```python
from build123d import *

# Parameters (mm, degrees)
F1_DEPTH = 1.524
F3_DEPTH = 40.132
F5_DEPTH = 2.794
F8_R     = 1.5875
F9_R     = 1.5875
F10_R    = 1.5875
F11_R    = 1.5875


with BuildPart() as f1:
    # F0 (on Right) → F1 (new body)
    with BuildSketch(Plane.YZ):
        with BuildLine():
            ThreePointArc((26.67, 16.002), (25.7400640303, 18.2470640303), (23.495, 19.177))
            Line((23.495, 19.177), (-23.495, 19.177))
            ThreePointArc((-23.495, 19.177), (-25.7400640303, 18.2470640303), (-26.67, 16.002))
            Line((-26.67, 16.002), (-26.67, -16.002))
            ThreePointArc((-26.67, -16.002), (-25.7400640303, -18.2470640303), (-23.495, -19.177))
            Line((-23.495, -19.177), (23.495, -19.177))
            ThreePointArc((23.495, -19.177), (25.7400640303, -18.2470640303), (26.67, -16.002))
            Line((26.67, -16.002), (26.67, 16.002))
        make_face()
    extrude(amount=F1_DEPTH)

    # F2 (on face) → F3 (join)
    with BuildSketch(Plane(origin=(0, 0, 0), x_dir=(0, -1, 0), z_dir=(-1, 0, 0))):
        with BuildLine():
            ThreePointArc((-23.495, 19.177), (-25.7400640303, 18.2470640303), (-26.67, 16.002))
            Line((-26.67, 16.002), (-26.67, -16.002))
            ThreePointArc((-26.67, -16.002), (-25.7400640303, -18.2470640303), (-23.495, -19.177))
            Line((-23.495, -19.177), (23.495, -19.177))
            ThreePointArc((23.495, -19.177), (25.7400640303, -18.2470640303), (26.67, -16.002))
            Line((26.67, -16.002), (26.67, 16.002))
            ThreePointArc((26.67, 16.002), (25.7400640303, 18.2470640303), (23.495, 19.177))
            Line((23.495, 19.177), (-23.495, 19.177))
        make_face()
        with BuildLine():
            ThreePointArc((25.146, -16.0655), (24.6810320151, -17.1880320151), (23.5585, -17.653))
            Line((23.5585, -17.653), (-23.5585, -17.653))
            ThreePointArc((-23.5585, -17.653), (-24.6810320151, -17.1880320151), (-25.146, -16.0655))
            Line((-25.146, -16.0655), (-25.146, 16.0655))
            ThreePointArc((-25.146, 16.0655), (-24.6810320151, 17.1880320151), (-23.5585, 17.653))
            Line((-23.5585, 17.653), (23.5585, 17.653))
            ThreePointArc((23.5585, 17.653), (24.6810320151, 17.1880320151), (25.146, 16.0655))
            Line((25.146, 16.0655), (25.146, -16.0655))
        make_face(mode=Mode.SUBTRACT)
    extrude(amount=F3_DEPTH)

    # F4 (on face) → F5 (join)
    with BuildSketch(Plane.YZ.offset(1.524)):
        with BuildLine():
            ThreePointArc((-26.67, 12.827), (-22.1798719395, 14.6868719395), (-20.32, 19.177))
            Line((-20.32, 19.177), (-23.495, 19.177))
            ThreePointArc((-23.495, 19.177), (-25.7400640303, 18.2470640303), (-26.67, 16.002))
            Line((-26.67, 16.002), (-26.67, 12.827))
        make_face()
    extrude(amount=F5_DEPTH)


with BuildPart() as f6_1:
    # F6: instance of F1
    add(f1.part.mirror(Plane.XY))


with BuildPart() as f1_1:
    add(f1.part)

    add(f6_1.part)  # F7 merges F6_1
    # F7: F6_1, F1 across plane
    add(f6_1.part.mirror(Plane.XZ))
    add(f1.part.mirror(Plane.XZ))

    # F8
    f8_edges = [f1_1.edges().sort_by_distance(p)[0] for p in [
        (1.524, -26.67, 0),
    ]]
    fillet(f8_edges, radius=F8_R)

    # F9
    f9_edges = [f1_1.edges().sort_by_distance(p)[0] for p in [
        (1.524, 0, -19.177),
    ]]
    fillet(f9_edges, radius=F9_R)

    # F10
    f10_edges = [f1_1.edges().sort_by_distance(p)[0] for p in [
        (1.524, 26.67, 0),
    ]]
    fillet(f10_edges, radius=F10_R)

    # F11
    f11_edges = [f1_1.edges().sort_by_distance(p)[0] for p in [
        (1.524, 0, 19.177),
    ]]
    fillet(f11_edges, radius=F11_R)


solid = f1_1.part
```
Input: part model. Units: mm. Frame: model coordinates. A direction names the side the tool comes from. Coordinates: 2 decimals unless noted, no trailing zeros. Loops run counter-clockwise (first coordinate to the right, second up) from the corner with the lowest first, then second, coordinate; pieces in that order, holes last.
Q1. Line query: line 1 along Z through (x, y) = (-1.5, 20); line 2 along Y through (x, z) = (-5, 2); line 3 along X through (y, z) = (-8, -2.5). Output: solid intervals per line, ascending.
Results are:
line 1: z = -19.18 to -17.65, 17.65 to 19.18
line 2: y = -26.67 to -25.15, 25.15 to 26.67
line 3: x = 0 to 1.52
Q2. Contact query for flat-ended pins moving along their axis: pin 1 (2 mm diameter, centred on y = 9, z = 9.5, fed in from +X); pin 2 (1 mm diameter, centred on y = -1.5, z = 0, fed in from -X). Output: stop coordinate, or through.
Results are:
pin 1: stops at x = 1.52
pin 2: stops at x = 0
Q3. Set-up query: faces 4 (the cylindrical face through (-18.218, 25.715, -18.272)), 5 (the flat face through (-20, 0, -17.653)), 6 (the cylindrical face through (2.58, 22.23, 14.64)). Return all of +Z, -Z, +X, -X, +Y, -Y with unobstructed straight access to the full face (end or side cutting, diameter ignored); none if empty.
Results are:
face 4: -Z, +X, -X, +Y
face 5: -X
face 6: +X
Q4. Mould query, pull axis Y, two halves, no side actions, for faces 1 (the cylindrical face through (-18.218, 25.715, 18.272)), 2 (the flat face through (-20, 25.146, 0)), 3 (the flat face through (-40.132, 0, -18)). Classes: +Y half, -Y half, draft (parallel to the pull), parting line (faces both ways), or undercut.
Results are:
face 1: +Y half
face 2: undercut
face 3: draft
Q5. Section C-C, the plane z = 1.5. Return the cut outline in (x, y) (1 decimal), and give its area (3 significant figures).
Results are:
outline: (-40.1, -26.7) - (-0.1, -26.7) arc R1.6 ccw to (1.5, -25.1) - (1.5, 25.1) arc R1.6 ccw to (-0.1, 26.7) - (-40.1, 26.7) - (-40.1, 25.1) - (0, 25.1) - (0, -25.1) - (-40.1, -25.1) - close
area: 203 mm2
Q6. Section D-D, the plane z = -15. Return the cut outline in (x, y).
Results are:
outline: (-40.13, -26.67) - (4.32, -26.67) - (4.32, -21.89) - (1.52, -21.89) - (1.52, 21.89) - (4.32, 21.89) - (4.32, 26.67) - (-40.13, 26.67) - (-40.13, 25.15) - (0, 25.15) - (0, -25.15) - (-40.13, -25.15) - close
Q7. Section B-B, the plane y = -16. Return the cut outline in (x, z) (1 decimal).
Results are:
outline: (-40.1, -19.2) - (-0.1, -19.2) arc R1.6 ccw to (1.5, -17.6) - (1.5, 17.6) arc R1.6 ccw to (-0.1, 19.2) - (-40.1, 19.2) - (-40.1, 17.7) - (0, 17.7) - (0, -17.7) - (-40.1, -17.7) - close
